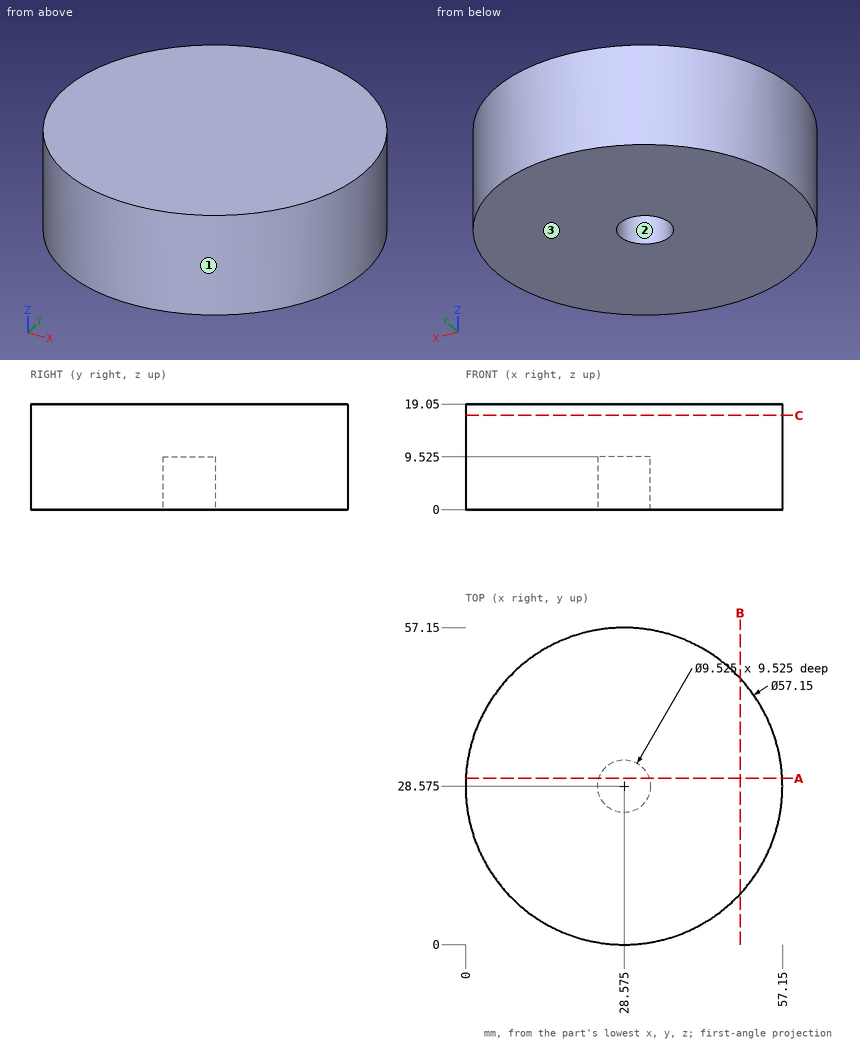
Geometry check sheet. Reference: drawing and pictorial views, mm from the part's lowest x, y, z. Give positions to 0.01 mm unless a question says otherwise; leave off trailing zeros. Loops run counter-clockwise (first coordinate to the right, second up) from the corner with the lowest first, then second, coordinate; pieces in that order, holes last. Notation, with made-up numbers: M 38,57 L 96,57 A7 ccw 96,64 Z; hole C 79,10 d5. An arc over 180 degrees is marked long. One line per question, with ' | ' between items.
Item 1: Depth check by flat-ended pin: P1, Ø2, axis at x = 7, z = 5, coming from the -Y side; P2, Ø10, axis at y = 50.5, z = 12, coming from the +X side; P3, Ø6, axis at x = 29, z = 9, coming from the +Y side. Enter the tip coordinate at first touch or a pass-through.
Completed:
P1: stops at y = 8.75 | P2: stops at x = 51.6 | P3: stops at y = 57.15
Item 2: Section check A-A, the plane y = 30. Record the cut outline in (x, z) (3 decimals), plus the area to 3 significant figures.
Completed:
outline: M 0.036,0 L 24.031,0 L 24.031,9.525 L 33.119,9.525 L 33.119,0 L 57.114,0 L 57.114,19.05 L 0.036,19.05 Z | area: 1,000 mm^2
Item 3: Section check B-B, the plane x = 49.5. Record the cut outline in (y, z), plus the area to 3 significant figures.
Completed:
outline: M 9.12,0 L 48.03,0 L 48.03,19.05 L 9.12,19.05 Z | area: 741 mm^2
Item 4: Draft check along X on the marked faces 1, 2 and 3. Enter one of: +X half, -X half, draft (parallel to the pull), parting line (faces both ways), or undercut.
Completed:
face 1: parting line | face 2: undercut | face 3: draft
Item 5: Thickness scan on line 1 (Y direction, x = 26, z = 7.5); line 2 (X direction, y = 40, z = 4.25); line 3 (Y direction, x = 34, z = 11.5). Record the ranges inside material, lowest first. Write a range as [from, to].
Completed:
line 1: y = [0.12, 24.57], [32.58, 57.03] | line 2: x = [2.38, 54.77] | line 3: y = [0.52, 56.63]
Item 6: Section check C-C, the plane z = 17. Record the cut outline in (x, y) (3 decimals), plus the area to 3 significant figures.
Completed:
outline: C 28.575,28.575 d57.15 | area: 2,570 mm^2
